Could you check a few things on this model? Use its own coordinates, in mm. Face numbers are marked on the shaded views. A direction names the side the tool comes from. Give positions to 0.01 mm unless a question says otherwise; leave off trailing zeros. Write each loop counter-clockwise with the first axis right and the second up, starting at its lowest first coordinate (ties: lowest second). Pieces come first, ordered by that corner, then holes. Notation, with made-up numbers: (28.5, 27) -> (66.5, 27) arc R17 cw to (66.5, 46) -> close; hole circle Ø8 at (83.25, 65.25). An arc over 180 degrees is marked (long way). One line per question, with ' | ' between items.
from build123d import *

# Parameters (mm, degrees)
F0_W      = 50
F0_H      = 50
F0_W_2    = 10
F0_H_2    = 10
F1_DEPTH  = 5
F2_DEPTH  = 75
F3_W      = 10
F3_H      = 5
F4_DEPTH  = 5
F5_W      = 10
F5_H      = 5
F6_DEPTH  = 5
F7_W      = 5
F7_H      = 10
F8_DEPTH  = 10
F10_D     = 6
F10_DEPTH = 20.001
F12_D     = 6
F13_R     = 4.99999
F14_DEPTH = 1
F15_DEPTH = 5
F16_SIZE  = 4.99999


# Not quite as in the source:
# - a fillet or chamfer is up to 0.001 mm smaller than in the source, because OpenCascade refuses the exact size


with BuildPart() as f1:
    # F0 (on Top) → F1 (new body)
    with BuildSketch(Plane.XY):
        Rectangle(F0_W, F0_H)
        Rectangle(F0_W_2, F0_H_2, mode=Mode.SUBTRACT)
    extrude(amount=F1_DEPTH)

    # F0 (on Top) → F2 (join)
    with BuildSketch(Plane.XY):
        Rectangle(F0_W_2, F0_H_2)
    extrude(amount=F2_DEPTH)

    # F3 (on face) → F4 (join)
    with BuildSketch(Plane.YZ.offset(5)):
        with Locations((0, 72.5)):
            Rectangle(F3_W, F3_H)
    extrude(amount=F4_DEPTH)

    # F5 (on face) → F6 (join)
    with BuildSketch(Plane(origin=(-5, 0, 0), x_dir=(0, -1, 0), z_dir=(-1, 0, 0))):
        with Locations((0, 72.5)):
            Rectangle(F5_W, F5_H)
    extrude(amount=F6_DEPTH)

    # F7 (on face) → F8 (join)
    with BuildSketch(Plane.XY.offset(75)):
        with Locations((7.5, 0)):
            Rectangle(F7_W, F7_H)
        with Locations((-7.5, 0)):
            Rectangle(F7_W, F7_H)
    extrude(amount=F8_DEPTH)

    # F10 (through all, one way)
    with BuildSketch(Plane(origin=(5, 0, 0), x_dir=(0, -1, 0), z_dir=(-1, 0, 0))):
        with Locations((0, 80)):
            Circle(F10_D / 2)
    extrude(amount=-F10_DEPTH, mode=Mode.SUBTRACT)

    # F12 (through all)
    with Locations(Plane.YZ.offset(-5)):
        with Locations((0, 80)):
            Hole(F12_D / 2)

    # F13 (radius 5 in the source; OpenCascade refuses exactly that, so slightly less here)
    f13_edges = [f1.edges().sort_by_distance(p)[0] for p in [
        (-7.5, -5, 85),
        (7.5, -5, 85),
        (7.5, 5, 85),
        (-7.5, 5, 85),
    ]]
    fillet(f13_edges, radius=F13_R)

    # F14 (cut): a face of the model
    f14_faces = [f1.faces().sort_by_distance(p)[0] for p in [
        (0, 0, 75),
    ]]
    extrude(f14_faces, amount=-F14_DEPTH, mode=Mode.SUBTRACT)

    # F15 (add): faces of the model
    f15_faces = [f1.faces().sort_by_distance(p)[0] for p in [
        (7.5, 0, 70),
        (-7.5, 0, 70),
    ]]
    extrude(f15_faces, amount=F15_DEPTH)

    # F16 (size 5 in the source; OpenCascade refuses exactly that, so slightly less here)
    f16_edges = [f1.edges().sort_by_distance(p)[0] for p in [
        (10, 0, 65),
        (-10, 0, 65),
    ]]
    chamfer(f16_edges, length=F16_SIZE)


solid = f1.part
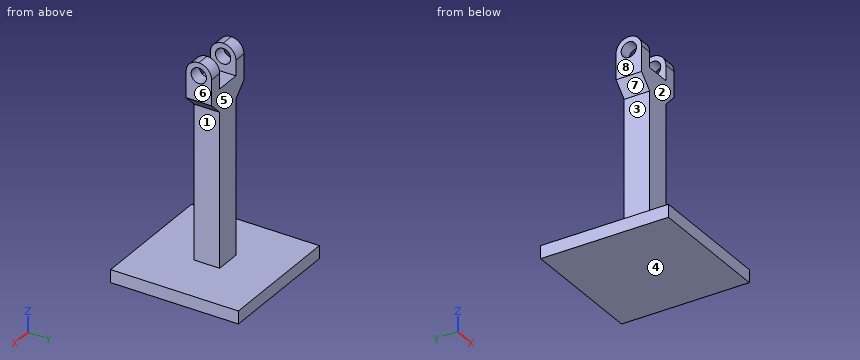
Q1. Imagine slicing it at D-D on x = -16. Please give me the cut outline in (y, z).
Answer below:
outline: (-25, 0) -> (25, 0) -> (25, 5) -> (-25, 5) -> close
Q2. Imagine slicing it at C-C on z = 30. Please give me the cut outline in (x, y), and give its area (3 significant figures).
Answer below:
outline: (-5, -5) -> (5, -5) -> (5, 5) -> (-5, 5) -> close | area: 100 mm^2
Q3. Imagine slicing it at A-A on x = 8. Count the separate pieces of the cut face and the enclosed holes in it, and give its area (3 significant figures).
Answer below:
separate pieces: 2 | enclosed holes: 1 | area: 381 mm^2
Q4. On a 3-axis mill with a long thin cutter (end or side, diameter ignored), from which of +Z, -Z, +X, -X, +Y, -Y can I reach the whole of each face in a straight line? I mean the marked faces 5, 6, 7 and 8. Say none if no direction works.
Answer below:
face 5: +Z, +X, -X, +Y | face 6: +Z, +X, +Y, -Y | face 7: -X, +Y, -Y | face 8: +Z, -X, +Y, -Y
Q5. Will these pins go through, and if not, where does the flat tip stop? pin 1 (1.5 mm diameter, centred on x = -19.5, y = 6.5, fed in from +Z); pin 2 (11 mm diameter, centred on y = 0.5, z = 22, fed in from -X); pin 3 (4 mm diameter, centred on y = -3.5, z = 52, fed in from +X); pin 4 (5.5 mm diameter, centred on y = 0, z = 80, fed in from -X).
Answer below:
pin 1: stops at z = 5 | pin 2: stops at x = -5 | pin 3: stops at x = 5 | pin 4: passes through
Q6. If we mould it in two halves opening along Z, with no side actions, what happens to the marked faces 1, 2, 3 and 4? For each: +Z half, -Z half, draft (parallel to the pull), parting line (faces both ways), or undercut.
Answer below:
face 1: undercut | face 2: draft | face 3: undercut | face 4: -Z half
Q7. If I drill on line 1 along Z through (x, y) = (-8, 0); line 2 along Z through (x, y) = (7.85, 0); line 3 along Z through (x, y) = (2.5, 2), over which ranges is the centre line in solid material (lowest first)?
Answer below:
line 1: z = 0 to 5, 68 to 77, 83 to 85 | line 2: z = 0 to 5, 67.85 to 77, 83 to 85 | line 3: z = 0 to 74
